For this review, take the finished solid that the model builds, in its own axes (mm). Face numbers are marked on the shaded views. Coordinates: 2 decimals unless noted, no trailing zeros. Loops run counter-clockwise (first coordinate to the right, second up) from the corner with the lowest first, then second, coordinate; pieces in that order, holes last.
1. To check wall thickness, follow probe 1 along Z at (x, y) = (0, -3.75); probe 2 along X at (y, z) = (-4.5, 5); probe 3 along Y at (x, z) = (0.25, 9.25). State the ranges of each line that lie inside material, in increasing order.
2. Take a section at A-A, the plane x = 0. State the section outline as (y, z) points.
3. Clearance check with a flat-ended pin moving along its axis: P1, Ø2, axis at x = -2, y = 0.5, coming from the +Z side. State where the tip first meets the part, or that it passes through.
4. Take a section at B-B, the plane z = 1.25. State the section outline as (x, y) points.
5. Mouldability with a two-part tool opening along X and no side actions: class the marked faces 1, 2 and 3 as pulls with the +X half, pulls with the -X half, needs draft (parallel to the pull), parting line crosses it, or undercut.
6. Take a section at C-C, the plane y = 1. State the section outline as (x, z) points, then the cut area to 3 significant figures.
7. Take a section at D-D, the plane y = -3.5. State the section outline as (x, z) points, then the cut area to 3 significant figures.
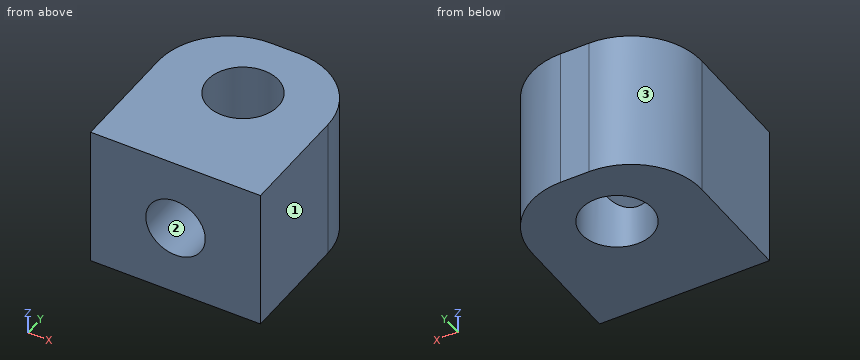
```python
from build123d import *

# Parameters (mm, degrees)
ESQUISSE1_W        = 12
ESQUISSE1_H        = 13
BOSS_EXTRU_1_DEPTH = 10
ESQUISSE3_W        = 2.5
ESQUISSE3_H        = 10
ESQUISSE4_W        = 2.1
ESQUISSE4_H        = 8
CONG_1_R           = 5


with BuildPart() as part:
    # Esquisse1 → Boss.-Extru.1 (new body)
    with BuildSketch(Plane(origin=(0, 0, 0), x_dir=(-1, 0, 0), z_dir=(0, 0, -1))):
        with Locations((0, -1.5)):
            Rectangle(ESQUISSE1_W, ESQUISSE1_H)
    extrude(amount=-BOSS_EXTRU_1_DEPTH)

    # Esquisse3 → Enlèvement de matière-Révolution1 (revolve, cut)
    with BuildSketch(Plane(origin=(0, 0, 0), x_dir=(1, 0, 0), z_dir=(0, 1, 0))):
        with Locations((1.25, -5)):
            Rectangle(ESQUISSE3_W, ESQUISSE3_H)
    revolve(axis=Axis((0, 0, 0), (0, 0, 1)), mode=Mode.SUBTRACT)

    # Esquisse4 → Diamètre du perçage Ø5.6 (5.6)1 (revolve, cut)
    with BuildSketch(Plane(origin=(0, 0, 5), x_dir=(0, 0, 1), z_dir=(1, 0, 0))):
        with Locations((1.05, 4)):
            Rectangle(ESQUISSE4_W, ESQUISSE4_H)
    revolve(axis=Axis((0, 6.35, 5), (0, -1, 0)), mode=Mode.SUBTRACT)

    # Congé1
    cong_1_edges = [part.edges().sort_by_distance(p)[0] for p in [
        (6, 5, 5),
        (-6, 5, 5),
    ]]
    fillet(cong_1_edges, radius=CONG_1_R)


solid = part.part
```
Results list:
1. probe 1: z = 0 to 2.9, 7.1 to 10
1. probe 2: x = -6 to -2.1, 2.1 to 6
1. probe 3: y = -8 to -2.49, 2.49 to 5
2. outline: (-8, 0) - (-2.5, 0) - (-2.5, 2.9) - (-8, 2.9) - close; (-8, 7.1) - (-2.5, 7.1) - (-2.5, 10) - (-8, 10) - close; (2.5, 0) - (5, 0) - (5, 10) - (2.5, 10) - close
3. P1: stops at z = 10
4. outline: (-6, -8) - (6, -8) - (6, 0) arc R5 ccw to (1, 5) - (-1, 5) arc R5 ccw to (-6, 0) - close; hole circle Ø5 at (0, 0)
5. face 1: pulls with the +X half
5. face 2: undercut
5. face 3: pulls with the -X half
6. outline: (-5.9, 0) - (-2.29, 0) - (-2.29, 10) - (-5.9, 10) - close; (2.29, 0) - (5.9, 0) - (5.9, 10) - (2.29, 10) - close
6. area: 72.2 mm2
7. outline: (-6, 0) - (6, 0) - (6, 10) - (-6, 10) - close; hole circle Ø4.2 at (0, 5)
7. area: 106 mm2
